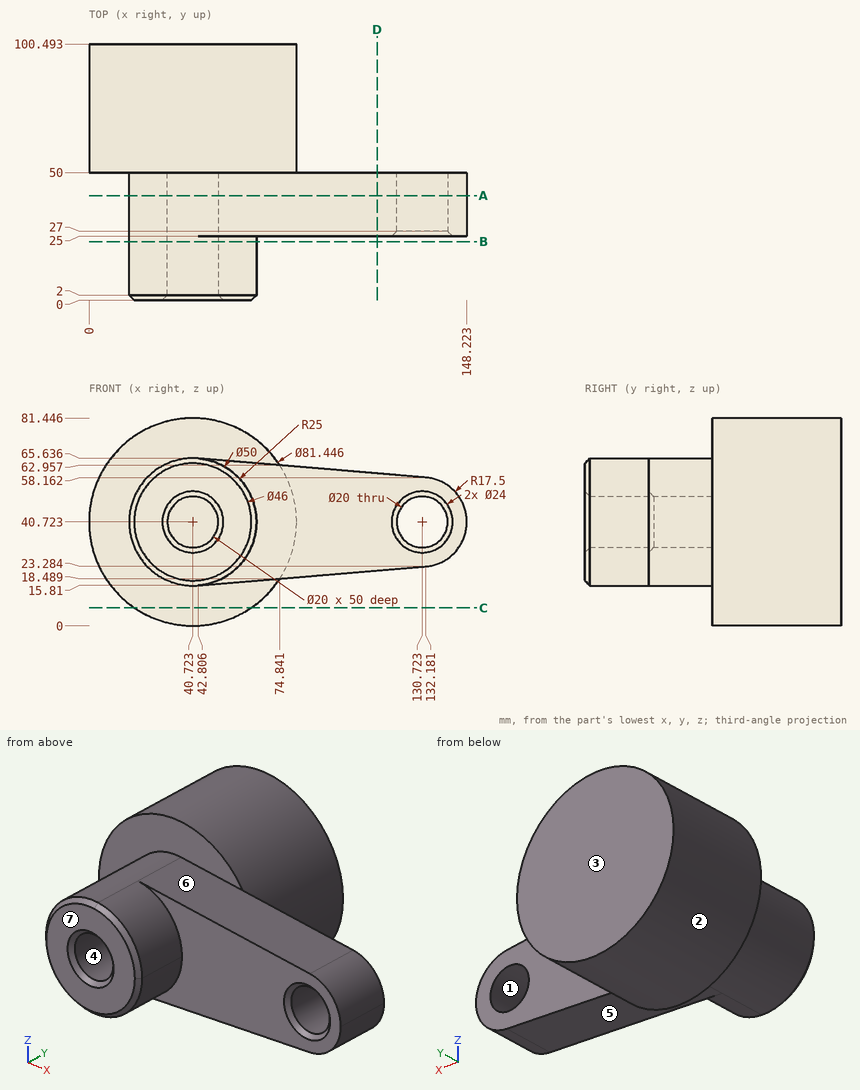
Geometry: see drawing. Coordinates: mm, zero at the bounding-box minimum. A direction names the side the tool comes from. Give positions to 0.01 mm unless a question says otherwise; leave off trailing zeros. Order: outer loops, then holes, each group sorted by start corner. A loop starts at its lowest first (then second) coordinate and runs counter-clockwise, first axis right, second up. Notation, with made-up numbers: (-20.75, 27.5) - (-11.75, 27.5) arc R16 ccw to (-11.75, 50.5) - close; hole circle Ø8 at (11, -16.75). An arc over 180 degrees is marked (long way). Write each question's results on one line, items separated by ' | '.
Item 1: Access query for the marked faces 5, 6 and 7. Directions: +Z, -Z, +X, -X, +Y, -Y. A direction counts if a zero-diameter tool reaches every point of the face in a straight line with its end or side. Return the directions, or none.
A:
face 5: -Z, +X, -Y | face 6: +Z, +X, -Y | face 7: +Z, -Z, +X, -X, -Y
Item 2: Section A-A (y = 41). Return loops of the section in (x, z), and give its area (3 significant figures).
A:
outline: (42.81, 15.81) - (132.18, 23.28) arc R17.5 ccw to (132.18, 58.16) - (42.81, 65.64) arc R25 ccw (long way) to start; hole circle Ø20 at (40.72, 40.72); hole circle Ø20 at (130.72, 40.72) | area: 4,670 mm^2
Item 3: Contact query for flat-ended pins moving along their axis: pin 1 Ø22 at (x, z) = (121.5, 36.5) entering from +Y; pin 2 Ø1 at (y, z) = (61.5, 66) entering from -X (1 decimal); pin 3 Ø15 at (x, z) = (81, 36) entering from -Y; pin 4 Ø18 at (x, z) = (130.72, 40.72) entering from +Y. Output: stop coordinate, or through.
A:
pin 1: stops at y = 50 | pin 2: stops at x = 8.4 | pin 3: stops at y = 25 | pin 4: passes through
Item 4: Material intervals for line 1 along X through (y, z) = (44, 41.5) (1 decimal); line 2 along X through (y, z) = (36.5, 35) (1 decimal); line 3 along Y through (x, z) = (47.5, 48), sorted ascending.
A:
line 1: x = 15.7 to 30.8, 50.7 to 120.8, 140.7 to 148.2 | line 2: x = 16.4 to 32.5, 48.9 to 122.5, 138.9 to 147.3 | line 3: y = 50 to 100.49
Item 5: Draft query along X for the marked faces 1, 2, 3 and 4. Return one class per face: released by +X, released by -X, zero draft, split by the parting line, or undercut.
A:
face 1: undercut | face 2: split by the parting line | face 3: zero draft | face 4: undercut
Item 6: Section D-D (x = 113). Return loops of the section in (y, z), and give its area (3 significant figures).
A:
outline: (25, 21.68) - (50, 21.68) - (50, 59.77) - (25, 59.77) - close | area: 952 mm^2
Item 7: Section C-C (z = 7). Return loops of the section in (x, y) (1 decimal), and give its area (3 significant figures).
A:
outline: (17.9, 50) - (63.6, 50) - (63.6, 100.5) - (17.9, 100.5) - close | area: 2,310 mm^2
Item 8: Section B-B (y = 23). Return loops of the section in (x, z).
A:
outline: (42.81, 15.81) arc R25 ccw to (65.72, 40.72) arc R25 ccw to (42.81, 65.64) arc R25 ccw (long way) to start; hole circle Ø20 at (40.72, 40.72)
